Print and shaded views of the part. All mm, measured from the part's lowest x, y and z. A direction names the side the tool comes from. Coordinates: 2 decimals unless noted, no trailing zeros. Order: outer loops, then holes, each group sorted by start corner. A loop starts at its lowest first (then second) coordinate and runs counter-clockwise, first axis right, second up. Notation, with made-up numbers: (52, 14.25) -> (77, 14.25) arc R11 ccw to (77, 30.25) -> close; hole circle Ø10 at (-14, -18.5). An arc over 180 degrees is marked (long way). Use one line per item in the form item = value. Start each with the question number.
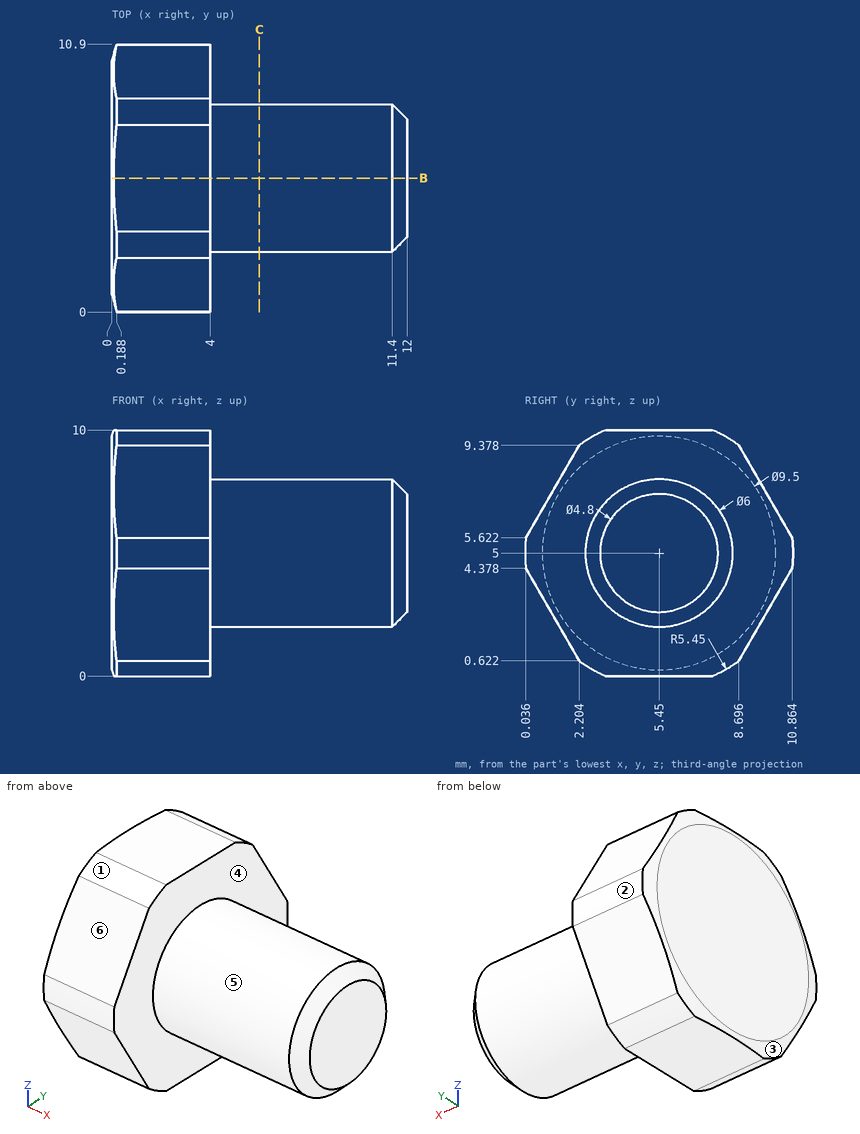
1) Cut at B-B on y = 5.45. Give the cut face in (x, z).
2) Probe L1, parallel to X at y = 10, z = 4; L2, parallel to Z at x = 3.25, y = 0.5 (1 decimal); L3, parallel to Z at x = 3.5, y = 10. List the from-to ranges inside material, lowest first.
3) Cut at C-C on x = 6. Give the cut face in (y, z), then the cut area to 3 significant figures.
4) Two-plate mould, pull along Y, no slides. Class the marked faces 1, 2, 3 and 4: released by +Y, released by -Y, zero draft, split by the parting line, or undercut.
5) Drop flat-ended pins along their axis: P1, Ø1.5, axis at x = 9.5, z = 3, coming from the +Y side; P2, Ø1, axis at y = 9.5, z = 1.5, coming from the -X side; P3, Ø2, axis at x = 8, z = 7.5, coming from the +Y side; P4, Ø2, axis at y = 5.5, z = 7.5, coming from the +X side. Give the stop position or say it passes through.
6) 3-axis set-ups, long thin cutter, end or side, ignore diameter. For the marked faces 5 and 6: which of +Z, -Z, +X, -X, +Y, -Y reach the whole face in a straight line?
Values follow:
q1.outline = (0, 0.25) -> (0.07, 0) -> (4, 0) -> (4, 2) -> (11.4, 2) -> (12, 2.6) -> (12, 7.4) -> (11.4, 8) -> (4, 8) -> (4, 10) -> (0.07, 10) -> (0, 9.75) -> close
q2.L1 = 0 to 4
q2.L2 = 3.6 to 6.4
q2.L3 = 2.88 to 7.12
q3.outline = circle Ø6 at (5.45, 5)
q3.area = 28.3 mm^2
q4.face_1 = released by -Y
q4.face_2 = released by +Y
q4.face_3 = split by the parting line
q4.face_4 = zero draft
q5.P1 = 8.18
q5.P2 = 0.03
q5.P3 = 8.05
q5.P4 = 12
q6.face_5 = +X
q6.face_6 = +Z, +X, -X, -Y
